The model under review builds one solid part; all positions refer to its coordinate system, in mm. Coordinates: 2 decimals unless noted, no trailing zeros. Order: outer loops, then holes, each group sorted by start corner. A loop starts at its lowest first (then second) coordinate and runs counter-clockwise, first axis right, second up.
Autodesk Fusion 360 part; units mm, degrees
sketch "スケッチ1" plane through (0, 0, 0) normal (0, 0, 1) x (1, 0, 0)
  line L0 (2.5, 186) -> (-92.5, 186)
  line L1 (-92.5, 186) -> (-92.5, -186)
  line L2 (-92.5, -186) -> (2.5, -186)
  line L3 (92.5, -30) -> (92.5, 180)
  line L4 (89.5161, 180) -> (-92.5, -186) construction
  line L5 (-92.5, 186) -> (53.8847, -108.352) construction
  line L6 (2.5, 186) -> (2.5, 180)
  line L7 (2.5, 180) -> (92.5, 180)
  line L8 (-92.5, -186) -> (2.5, -186) construction
  line L9 (92.5, -50) -> (2.5, -186)
  line L10 (92.5, -50) -> (2.5, -50)
  line L11 (2.5, -50) -> (2.5, -30)
  line L12 (2.5, -30) -> (92.5, -30)
  dimension "d2" = 372
  dimension "d5" = 95
  dimension "d7" = 90
  dimension "d8" = 20
extrude "押し出し1" add sketch "スケッチ1" along normal blind 6
chamfer "面取り1" distance 30 angle 45 2 edges at (-92.5, -186, 3) (-92.5, 186, 3)
sketch "スケッチ2" plane through (0, 0, 6) normal (0, 0, 1) x (-1, 0, 0)
  line L0 (62.5, -186) -> (92.5, -156)
  line L1 (92.5, -156) -> (92.5, 156)
  line L2 (92.5, 156) -> (62.5, 186)
  line L3 (62.5, 186) -> (-2.5, 186)
  line L4 (-2.5, 186) -> (-92.5, 50)
  line L5 (-92.5, 50) -> (-2.5, 50)
  line L6 (-2.5, 50) -> (-2.5, 30)
  line L7 (-2.5, 30) -> (-92.5, 30)
  line L8 (-92.5, 30) -> (-92.5, -180)
  line L9 (-92.5, -180) -> (-2.5, -180)
  line L10 (-2.5, -180) -> (-2.5, -186)
  line L11 (-2.5, -186) -> (62.5, -186)
  line L12 (-92.5, -180) -> (-52.5, -180) construction
  line L13 (-52.5, -180) -> (-52.5, -135) construction
  line L14 (-52.5, -135) -> (-92.5, -135) construction
  line L15 (-92.5, -135) -> (-92.5, -180) construction
  line L16 (-52.5, -135) -> (-52.5, -75) construction
  line L17 (-52.5, -75) -> (-52.5, -15) construction
  point P0 (-52.5, -135)
  point P1 (-52.5, -75)
  dimension "d12" = 40
  dimension "d13" = 45
  dimension "d14" = 60
  dimension "d15" = 60
hole "穴1" at (52.5, 135, 6) at (52.5, 75, 6) at (52.5, 15, 6) direction (0, 0, -1) diameter 18 end through all
equation "d5 = 30 mm + 65 mm"
(1) Consider section A-A (z = 4.55). Give the boundary of the cut face in (x, y), then the cut area to 3 significant figures.
(2) Insertion check: pin 1 Ø1 at (x, z) = (72, 2) entering from -Y; pin 2 Ø1.8 at (x, z) = (47, 4) entering from +Y; pin 3 Ø1 at (x, z) = (-70.5, 3) entering from -Y. Each pin has a flat end and moves straight along its axis. Give the tip position at first contact, or say it passes through.
(3) Wall thickness on line 1 (X direction, y = 135, z = 3.85); line 2 (Y direction, x = 52.5, z = 1.25); line 3 (Y direction, x = 83, z = 4.05): over which ranges is each line inside the solid? List them lowest first.
(4) Consider section C-C (x = 22). Give the boundary of the cut face in (y, z), then the cut area to 3 significant figures.
(5) The part is to be moulded in two halves that separate along Y. For faces 1 (the face through (48.13, -117.05, 2.96)), 2 (the face through (-1, 3, 0)), 3 (the face through (49.797, 66.416, 2.958)), say which applies: +Y half, -Y half, draft (parallel to the pull), parting line (faces both ways), or undercut.
(6) Consider section D-D (x = 52.5). Give the boundary of the cut face in (y, z).
(7) Consider section B-B (y = 75). Give the boundary of the cut face in (x, z).
Findings:
1. outline: (-92.5, -156) - (-62.5, -186) - (2.5, -186) - (92.5, -50) - (2.5, -50) - (2.5, -30) - (92.5, -30) - (92.5, 180) - (2.5, 180) - (2.5, 186) - (-62.5, 186) - (-92.5, 156) - close; hole circle Ø18 at (52.5, 15); hole circle Ø18 at (52.5, 75); hole circle Ø18 at (52.5, 135)
1. area: 58,700 mm2
2. pin 1: stops at y = -81.73
2. pin 2: stops at y = 180
2. pin 3: stops at y = -178.5
3. line 1: x = -92.5 to 43.5, 61.5 to 92.5
3. line 2: y = -110.44 to -50, -30 to 6, 24 to 66, 84 to 126, 144 to 180
3. line 3: y = -64.36 to -50, -30 to 180
4. outline: (-156.53, 0) - (-50, 0) - (-50, 6) - (-156.53, 6) - close; (-30, 0) - (180, 0) - (180, 6) - (-30, 6) - close
4. area: 1,900 mm2
5. face 1: -Y half
5. face 2: draft
5. face 3: undercut
6. outline: (-110.44, 0) - (-50, 0) - (-50, 6) - (-110.44, 6) - close; (-30, 0) - (6, 0) - (6, 6) - (-30, 6) - close; (24, 0) - (66, 0) - (66, 6) - (24, 6) - close; (84, 0) - (126, 0) - (126, 6) - (84, 6) - close; (144, 0) - (180, 0) - (180, 6) - (144, 6) - close
7. outline: (-92.5, 0) - (43.5, 0) - (43.5, 6) - (-92.5, 6) - close; (61.5, 0) - (92.5, 0) - (92.5, 6) - (61.5, 6) - close
